Autodesk Inventor part; units mm, degrees
ref_plane "YZ Plane" through (0, 0, 0) normal (1, 0, 0) x (0, 1, 0)
ref_plane "XZ Plane" through (0, 0, 0) normal (0, 1, 0) x (-1, 0, 0)
ref_plane "XY Plane" through (0, 0, 0) normal (0, 0, 1) x (1, 0, 0)
sketch "Sketch1" plane through (0, 0, 0) normal (0, 0, 1) x (1, 0, 0)
  line L0 (0, 0) -> (25.4, 0)
  line L1 (25.4, 0) -> (25.4, 50.8)
  line L2 (25.4, 50.8) -> (0, 50.8)
  line L3 (0, 50.8) -> (0, 0)
  line L4 (3.175, 47.625) -> (22.225, 47.625)
  line L5 (22.225, 47.625) -> (22.225, 3.175)
  line L6 (22.225, 3.175) -> (3.175, 3.175)
  line L7 (3.175, 3.175) -> (3.175, 47.625)
  dimension "d0" = 25.4
  dimension "d1" = 50.8
  dimension "d2" = 3.175
extrude "Beam" add sketch "Sketch1" along normal mid plane 469.9
sketch "Sketch2" plane through (0, 50.8, -234.95) normal (0, 1, 0) x (1, 0, 0)
  line L0 (0, 0) -> (25.4, 0)
  line L1 (0, 0) -> (0, -469.9)
  point P0 (6.35, -6.35)
  dimension "d5" = 6.35
  dimension "d6" = 6.35
hole "Rivet Hole" at (6.35, 50.8, -228.6) direction (0, -1, 0) diameter 3.175 end up to surface
pattern_linear "Rivet Holes" count 2 spacing 12.7 along (1, 0, 0) count 2 spacing 12.7 along (0, 0, 1) of "Rivet Hole"
mirror "Rivet Holes Mirrored" about plane through (0, 0, 0) normal (0, 0, 1) of "Rivet Hole", "Rivet Holes"
properties part number "Back Beam"
For this review, take the finished solid that the model builds, in its own axes (mm). A direction names the side the tool comes from. Round coordinates to 2 decimals unless told otherwise and drop trailing zeros. Order: outer loops, then holes, each group sorted by start corner. A loop starts at its lowest first (then second) coordinate and runs counter-clockwise, first axis right, second up.
Q1. We need section A-A, the plane y = 30. Give the boundary of the cut face in (x, z) (3 decimals).
Findings below:
outline: (0, -234.95) - (3.175, -234.95) - (3.175, 234.95) - (0, 234.95) - close; (22.225, -234.95) - (25.4, -234.95) - (25.4, 234.95) - (22.225, 234.95) - close
Q2. Wall thickness on line 1 (X direction, y = 49.85, z = 228.6); line 2 (Z direction, x = 6.35, y = 48.55); line 3 (Y direction, x = 14.25, z = 36) (3 decimals): over which ranges is each line inside the solid? List them lowest first.
Findings below:
line 1: x = 0 to 4.76, 7.94 to 17.46, 20.64 to 25.4
line 2: z = -234.95 to -230.19, -227.01 to -217.49, -214.31 to 214.31, 217.49 to 227.01, 230.19 to 234.95
line 3: y = 0 to 3.175, 47.625 to 50.8
Q3. We need section B-B, the plane z = -94.5. Give the boundary of the cut face in (x, y) (3 decimals), plus the area to 3 significant figures.
Findings below:
outline: (0, 0) - (25.4, 0) - (25.4, 50.8) - (0, 50.8) - close; hole (3.175, 3.175) - (22.225, 3.175) - (22.225, 47.625) - (3.175, 47.625) - close
area: 444 mm2
Q4. Machinability: for faces 4 (the flat face through (2, 24, -234.95)), 5 (the flat face through (22.225, 26, -3)), which of the approach directions +Z, -Z, +X, -X, +Y, -Y give a long, thin tool a straight path to every point of the face, cutting with its end or side? Answer none if there is none.
Findings below:
face 4: -Z, +X, -X, +Y, -Y
face 5: +Z, -Z
Q5. Insertion check: P1, Ø3, axis at x = 19.05, z = -228.6, coming from the +Y side (3 decimals). The pin has a flat end and moves straight along its axis. Give the tip position at first contact, or say it passes through.
Findings below:
P1: stops at y = 3.175
Q6. Mouldability with a two-part tool opening along Y and no side actions: class faces 1 (the flat face through (13, 3.175, -3)), 2 (the flat face through (13, 50.8, -3)), 3 (the flat face through (0, 26, -3)) as pulls with the +Y half, pulls with the -Y half, needs draft (parallel to the pull), parting line crosses it, or undercut.
Findings below:
face 1: undercut
face 2: pulls with the +Y half
face 3: needs draft
